Build history of the part. All positions in model axes, mm. A direction names the side the tool comes from. Round coordinates to 2 decimals unless told otherwise and drop trailing zeros. Loops run counter-clockwise (first coordinate to the right, second up) from the corner with the lowest first, then second, coordinate; pieces in that order, holes last. Notation, with made-up numbers: (-34, 57.5) - (-11, 57.5) arc R13 cw to (-11, 65.5) - close; hole circle Ø3 at (21, -24.75). An arc over 180 degrees is marked (long way). Use a Markdown table: item, result.
from build123d import *


with BuildPart() as part:
    # 草图1 → 旋转1 (revolve)
    with BuildSketch(Plane.XY, mode=Mode.PRIVATE) as revolve_1_sk:
        with BuildLine():
            Line((-4.838882373, 3.10342775), (-5.028769085, 0.933012702))
            Line((-5.028769085, 0.933012702), (-5.528769085, 0.933012702))
            Line((-5.528769085, 0.933012702), (-5.778769085, 0.5))
            Line((-5.778769085, 0.5), (-10, 0.5))
            Line((-10, 0.5), (-10, 6.5))
            Line((-10, 6.5), (-5.528769085, 6.5))
            Line((-5.528769085, 6.5), (-5.528769085, 7))
            Line((-5.528769085, 7), (-10.5, 7))
            Line((-10.5, 7), (-11, 6.5))
            Line((-11, 6.5), (-11, 0.5))
            Line((-11, 0.5), (-10.5, 0))
            Line((-10.5, 0), (-5.0084872, 0))
            ThreePointArc((-5.0084872, 0), (-4.6084872, 0.3), (-4.2084872, 0))
            Line((-4.2084872, 0), (-3.340059177, 0.075977607))
            Line((-3.340059177, 0.075977607), (-4.564742869, 0.5))
            Line((-4.564742869, 0.5), (-4.389765542, 2.5))
            Line((-4.389765542, 2.5), (-3.340059177, 2.5))
            Line((-3.340059177, 2.5), (-3, 4.428571429))
            Line((-3, 4.428571429), (-3.918095147, 5.071428571))
            Line((-3.918095147, 5.071428571), (-5.038882373, 5.071428571))
            Line((-5.038882373, 5.071428571), (-5.038882373, 3.950641346))
            ThreePointArc((-5.038882373, 3.950641346), (-5.274132553, 3.447892716), (-4.838882373, 3.10342775))
        make_face()
    revolve(revolve_1_sk.sketch.rotate(Axis((0, 0, 0), (0, 1, 0)), 270), axis=Axis((0, 0, 0), (0, 1, 0)))


solid = part.part
Q1. Cut at A-A, the plane y = 1.5. List the corners of the cut face in (x, z), plus the area to 3 significant figures.
Results found:
| item | result |
|---|---|
| outline | circle Ø22 at (0, 0); circle Ø9.96 at (0, 0); hole circle Ø20 at (0, 0); hole circle Ø8.95 at (0, 0) |
| area | 80.9 mm2 |
Q2. Which spindle directions (+Z, -Z, +X, -X, +Y, -Y) get a long thin tool onto all of the face, cutting with end or side? Do faces 1 (the face through (5.397, 6.754, 1.199)), 2 (the face through (2.7, 1.96, 3.52)), 3 (the face through (1.858, 4.121, 2.424)). Say none if no direction does.
Results found:
| item | result |
|---|---|
| face 1 | +Y |
| face 2 | none |
| face 3 | -Y |
Q3. Pull direction Z, two halves, no side cores. Call faces 4 (the face through (4.3, 0.5, 4.3)), 5 (the face through (5, 7, 5)), 6 (the face through (10.74, 3.46, 2.38)): pulls with the +Z half, pulls with the -Z half, needs draft (parallel to the pull), parting line crosses it, or undercut.
Results found:
| item | result |
|---|---|
| face 4 | undercut |
| face 5 | needs draft |
| face 6 | parting line crosses it |
Q4. Probe line 1 (X direction, y = 2, z = 0.25); line 2 (Y direction, x = 2.5, z = 8.5); line 3 (Z direction, x = -4, y = 4.5). List the from-to ranges inside material, lowest first.
Results found:
| item | result |
|---|---|
| line 1 | x = -11 to -10, -4.93 to -4.43, 4.43 to 4.93, 10 to 11 |
| line 2 | y = 0 to 0.5, 6.5 to 7 |
| line 3 | z = -10.25 to -9.17, -3.06 to 3.06, 9.17 to 10.25 |
Q5. Cut at B-B, the plane y = 3.5. List the corners of the cut face in (x, z), plus the area to 3 significant figures.
Results found:
| item | result |
|---|---|
| outline | circle Ø22 at (0, 0); circle Ø10.57 at (0, 0); hole circle Ø20 at (0, 0); hole circle Ø6.33 at (0, 0) |
| area | 122 mm2 |
Q6. Drop flat-ended pins along their axis: pin 1 (3 mm diameter, centred on x = 5, y = 4, fed in from +Z); pin 2 (3 mm diameter, centred on x = 2, z = 1.5, fed in from +Y); pin 3 (5 mm diameter, centred on x = 1, z = -0.5, fed in from -Y). Give the stop position or say it passes through.
Results found:
| item | result |
|---|---|
| pin 1 | stops at z = 10.43 |
| pin 2 | stops at y = 5.07 |
| pin 3 | stops at y = 0.05 |
